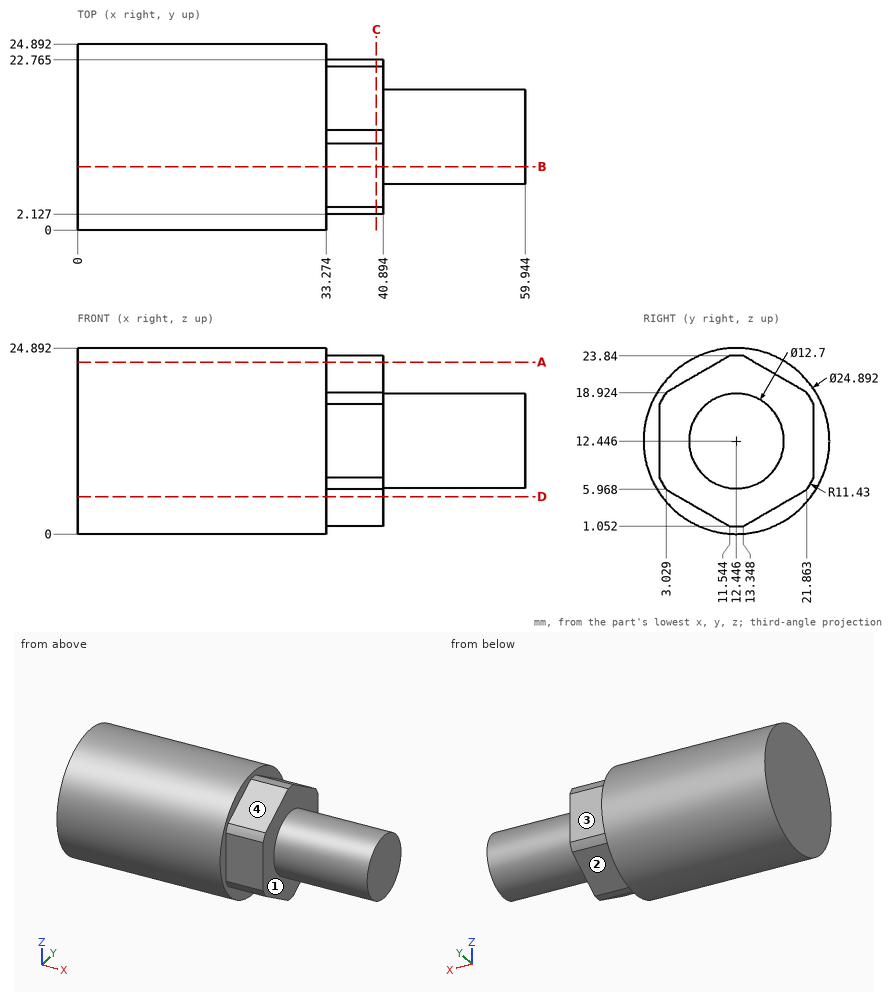
Could you check a few things on this drawing? It's one solid part, dimensions in mm from its lowest x, y, z. A direction names the side the tool comes from. Coordinates: 2 decimals unless noted, no trailing zeros. Order: outer loops, then holes, each group sorted by start corner. A loop starts at its lowest first (then second) coordinate and runs counter-clockwise, first axis right, second up.
1. For the marked faces 1, 2, 3 and 4, which set-ups out of +Z, -Z, +X, -X, +Y, -Y let a thin tool reach every point of the face, with its end or its side?
2. I need wall thicknesses on line 1 (X direction, y = 2, z = 6); line 2 (X direction, y = 20.5, z = 11.75); line 3 (Y direction, x = 26, z = 7) (1 decimal). Which ranges of each line are inside material? Lowest first, please.
3. If we section it at A-A (z = 23): Please give me the cut outline in (x, y).
4. If we section it at D-D (z = 5): Please give me the cut outline in (x, y) (1 decimal).
5. I'm going to push flat-ended pins straight in: pin 1 (1.5 mm diameter, centred on y = 5, z = 6, fed in from +X); pin 2 (1.5 mm diameter, centred on x = 36.5, y = 19.5, fed in from -Z); pin 3 (8 mm diameter, centred on x = 48, z = 11.5, fed in from +Y). Where does each tip first touch, or does it pass through?
6. If we section it at B-B (y = 8.5): Please give me the cut outline in (x, z), then the cut area to 3 significant figures.
7. If we section it at C-C (x = 40): Please give me the cut outline in (y, z) (1 decimal), then the cut area to 3 significant figures.
Entries:
1. face 1: +X
1. face 2: -Z, +X, +Y
1. face 3: +Z, -Z, +X, +Y
1. face 4: +Z, +X, -Y
2. line 1: x = 0 to 33.27
2. line 2: x = 0 to 40.89
2. line 3: y = 1.3 to 23.6
3. outline: (0, 5.85) - (33.27, 5.85) - (33.27, 10.09) - (40.89, 10.09) - (40.89, 14.8) - (33.27, 14.8) - (33.27, 19.04) - (0, 19.04) - close
4. outline: (0, 2.5) - (33.3, 2.5) - (33.3, 4.7) - (40.9, 4.7) - (40.9, 20.2) - (33.3, 20.2) - (33.3, 22.4) - (0, 22.4) - close
5. pin 1: stops at x = 40.89
5. pin 2: stops at z = 4.17
5. pin 3: stops at y = 18.8
6. outline: (0, 0.64) - (33.27, 0.64) - (33.27, 2.81) - (40.89, 2.81) - (40.89, 7.47) - (59.94, 7.47) - (59.94, 17.42) - (40.89, 17.42) - (40.89, 22.08) - (33.27, 22.08) - (33.27, 24.25) - (0, 24.25) - close
6. area: 1,120 mm2
7. outline: (2.1, 7.5) arc R11.4 ccw to (3, 6) - (11.5, 1.1) arc R11.4 ccw to (13.3, 1.1) - (21.9, 6) arc R11.4 ccw to (22.8, 7.5) - (22.8, 17.4) arc R11.4 ccw to (21.9, 18.9) - (13.3, 23.8) arc R11.4 ccw to (11.5, 23.8) - (3, 18.9) arc R11.4 ccw to (2.1, 17.4) - close
7. area: 366 mm2
